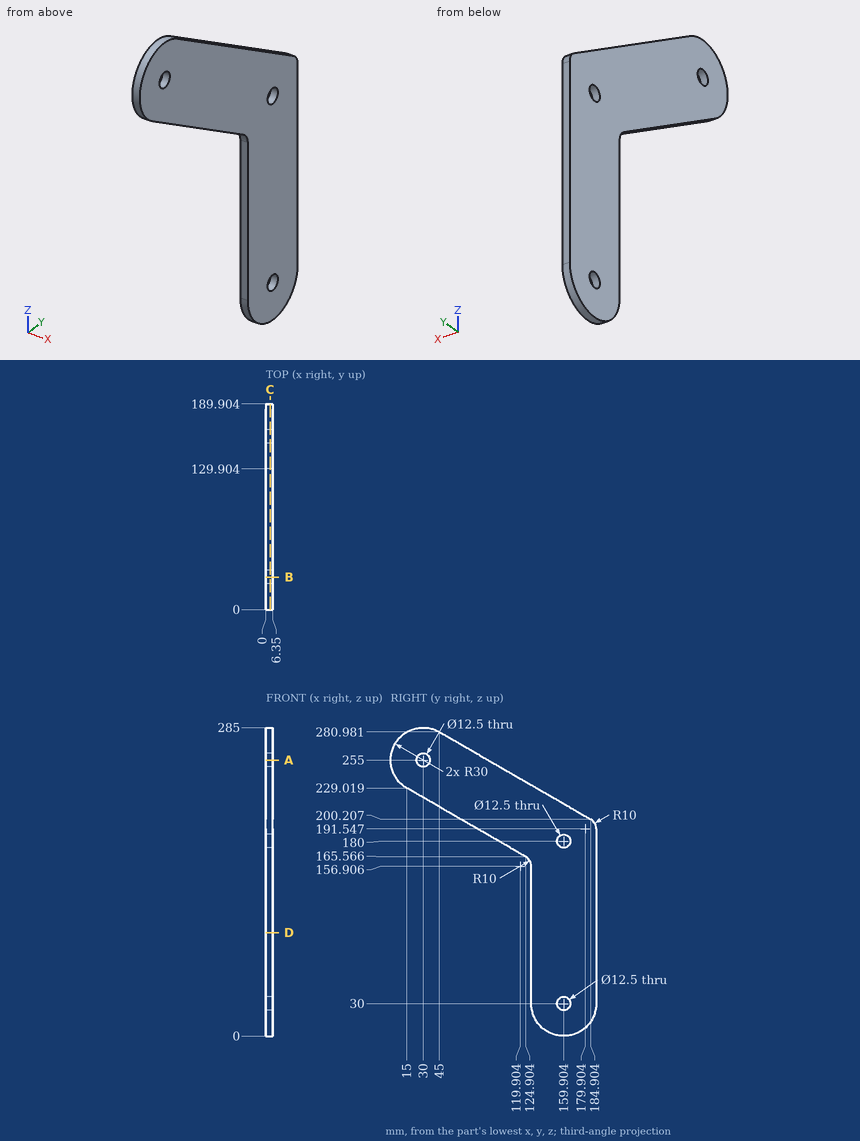
For this review, use the dimensioned drawing (mm, ordinates from the lowest corner) and the shaded views. Round coordinates to 2 decimals unless told otherwise and drop trailing zeros. Loops run counter-clockwise (first coordinate to the right, second up) from the corner with the lowest first, then second, coordinate; pieces in that order, holes last. Notation, with made-up numbers: M 89.25,5 L 116.25,5 A18 cw 116.25,17 Z; hole C -28.5,24 d11. An arc over 180 degrees is marked long. Answer as a JSON object with one key per item and string values.
(1) Clearance check with flat-ended pins moving along their axes: P1, Ø1, axis at x = 3.5, y = 82, coming from the +Z side; P2, Ø2, axis at x = 3, y = 61.5, coming from the +Z side; P3, Ø3, axis at x = 1.5, z = 69.5, coming from the -Y side. State where each tip first meets the part, or that it passes through.
Resolved:
{"P1": "z = 259.91", "P2": "z = 272.03", "P3": "y = 129.9"}
(2) Take a section at C-C on x = 4. Give the boundary of the cut face in (y, z).
Resolved:
{"outline": "M 15,229.02 L 124.9,165.57 A10 cw 129.9,156.91 L 129.9,30 A30 ccw 189.9,30 L 189.9,191.55 A10 ccw 184.9,200.21 L 45,280.98 A30 ccw Z; hole C 30,255 d12.5; hole C 159.9,30 d12.5; hole C 159.9,180 d12.5"}
(3) Take a section at A-A on z = 255. Give the boundary of the cut face in (x, y).
Resolved:
{"outline": "M 0,0 L 6.35,0 L 6.35,23.75 L 0,23.75 Z; M 0,36.25 L 6.35,36.25 L 6.35,90 L 0,90 Z"}
(4) To check wall thickness, follow line 1 along Y through (x, z) = (1.5, 97); line 2 along Y through (x, z) = (2.75, 180) (1 decimal); line 3 along Y through (x, z) = (5, 255). State the ranges of each line that lie inside material, in increasing order.
Resolved:
{"line 1": "129.9 to 189.9", "line 2": "99.9 to 153.7, 166.2 to 189.9", "line 3": "0 to 23.75, 36.25 to 90"}
(5) Take a section at B-B on y = 30. Give the boundary of the cut face in (x, z).
Resolved:
{"outline": "M 0,220.36 L 6.35,220.36 L 6.35,248.75 L 0,248.75 Z; M 0,261.25 L 6.35,261.25 L 6.35,285 L 0,285 Z"}
(6) Take a section at D-D on z = 95.5. Give the boundary of the cut face in (x, y), and give its area (3 significant figures).
Resolved:
{"outline": "M 0,129.9 L 6.35,129.9 L 6.35,189.9 L 0,189.9 Z", "area": "381 mm²"}
